Could you check a few things on this model? Use its own coordinates, in mm. A direction names the side the tool comes from. Give positions to 0.01 mm unless a question says otherwise; leave off trailing zeros. Loops run counter-clockwise (first coordinate to the right, second up) from the corner with the lowest first, then second, coordinate; pieces in that order, holes last. Notation, with made-up numbers: (53.25, 47.5) - (71.25, 47.5) arc R27 cw to (71.25, 77.5) - close; hole circle Ø10 at (32, 61.5). An arc over 180 degrees is marked (long way). Use CSV: the item, a comma, the result in double quotes.
from build123d import *

# Parameters (mm, degrees)
SKETCH_R           = 4.25
PAD_DEPTH          = 10
SKETCH001_W        = 16
SKETCH001_H        = 16
POCKET_DEPTH       = 5
FILLET_R           = 7
SKETCH002_W        = 180
SKETCH002_H        = 180
SKETCH002_R        = 57.5
SKETCH002_R_2      = 8
PAD001_DEPTH       = 10
SKETCH003_R        = 58.25
POCKET001_DEPTH    = 20.0010001
SKETCH004_W        = 30
SKETCH004_H        = 30
SKETCH004_R        = 5.5
SKETCH004_R_2      = 1.75
PAD002_DEPTH       = 10
SKETCH005_R        = 12.5
POCKET002_DEPTH    = 5
FILLET001_R        = 14.99
FILLET001_FACE62_R = 4.25
POCKET003_DEPTH    = 10.001
POCKET004_DEPTH    = 10
FILLET002_R        = 7


with BuildPart() as part:
    # Sketch → Pad (new body)
    with BuildSketch(Plane.XY):
        with BuildLine():
            ThreePointArc((0, -57.5), (57.5, 0), (0, 57.5))
            Line((0, 64.5658578507), (0, 57.5))
            Line((-7.5, 64.5658578507), (0, 64.5658578507))
            Line((-7.5, 79.5658578507), (-7.5, 64.5658578507))
            Line((7.5, 79.5658578507), (-7.5, 79.5658578507))
            Line((7.5, 64.5658578507), (7.5, 79.5658578507))
            ThreePointArc((7, -64.6219776856), (64.9995131723, -0.2515697895), (7.5, 64.5658578507))
            Line((7, -64.6219776856), (7, -79.6219776856))
            Line((7, -79.6219776856), (0, -79.6219776856))
            Line((0, -79.6219776856), (0, -57.5))
        make_face()
        with Locations((0, 72.0658578507)):
            Circle(SKETCH_R, mode=Mode.SUBTRACT)
    extrude(amount=PAD_DEPTH)

    # Sketch001 (on Face13 of Pad) → Pocket (cut)
    with BuildSketch(Plane.XY.offset(10)):
        with Locations((-0.5, 72.5)):
            Rectangle(SKETCH001_W, SKETCH001_H)
    extrude(amount=-POCKET_DEPTH, mode=Mode.SUBTRACT)

    # Fillet
    fillet_edges = [part.edges().sort_by_distance(p)[0] for p in [
        (-7.5, 64.565858, 2.5),
        (-7.5, 79.565858, 2.5),
    ]]
    fillet(fillet_edges, radius=FILLET_R)

    # Sketch002 → Pad001 (join)
    with BuildSketch(Plane.XY):
        Rectangle(SKETCH002_W, SKETCH002_H)
        Circle(SKETCH002_R, mode=Mode.SUBTRACT)
        with Locations((75, -75)):
            Circle(SKETCH002_R_2, mode=Mode.SUBTRACT)
        with Locations((75, 75)):
            Circle(SKETCH002_R_2, mode=Mode.SUBTRACT)
        with Locations((-75, 75)):
            Circle(SKETCH002_R_2, mode=Mode.SUBTRACT)
        with Locations((-75, -75)):
            Circle(SKETCH002_R_2, mode=Mode.SUBTRACT)
    extrude(amount=-PAD001_DEPTH)

    # Sketch003 (on Face26 of Pad001) → Pocket001 (cut, through all)
    with BuildSketch(Plane(origin=(0, 0, -10), x_dir=(1, 0, 0), z_dir=(0, 0, -1))):
        Circle(SKETCH003_R)
    extrude(amount=-POCKET001_DEPTH, mode=Mode.SUBTRACT)

    # Sketch004 (on Face2 of Pocket001) → Pad002 (join)
    with BuildSketch(Plane.XY):
        with Locations((0, 105)):
            Rectangle(SKETCH004_W, SKETCH004_H)
        with Locations((0, 105)):
            Circle(SKETCH004_R, mode=Mode.SUBTRACT)
        with Locations((8, 105)):
            Circle(SKETCH004_R_2, mode=Mode.SUBTRACT)
        with Locations((0, 113)):
            Circle(SKETCH004_R_2, mode=Mode.SUBTRACT)
        with Locations((-8, 105)):
            Circle(SKETCH004_R_2, mode=Mode.SUBTRACT)
        with Locations((0, 97)):
            Circle(SKETCH004_R_2, mode=Mode.SUBTRACT)
        with Locations((0, -105)):
            Rectangle(SKETCH004_W, SKETCH004_H)
        with Locations((0, -105)):
            Circle(SKETCH004_R, mode=Mode.SUBTRACT)
        with Locations((8, -105)):
            Circle(SKETCH004_R_2, mode=Mode.SUBTRACT)
        with Locations((0, -97)):
            Circle(SKETCH004_R_2, mode=Mode.SUBTRACT)
        with Locations((-8, -105)):
            Circle(SKETCH004_R_2, mode=Mode.SUBTRACT)
        with Locations((0, -113)):
            Circle(SKETCH004_R_2, mode=Mode.SUBTRACT)
    extrude(amount=-PAD002_DEPTH)

    # Sketch005 (on Face13 of Pad002) → Pocket002 (cut)
    with BuildSketch(Plane.XY):
        with Locations((0, 105)):
            Circle(SKETCH005_R)
        with Locations((0, -105)):
            Circle(SKETCH005_R)
    extrude(amount=-POCKET002_DEPTH, mode=Mode.SUBTRACT)

    # Fillet001
    fillet001_edges = [part.edges().sort_by_distance(p)[0] for p in [
        (15, -120, -5),
        (-15, -120, -5),
        (15, -90, -5),
        (-15, -90, -5),
        (15, 120, -5),
        (-15, 120, -5),
        (15, 90, -5),
        (-15, 90, -5),
        (90, 90, -5),
        (90, -90, -5),
        (-90, -90, -5),
        (-90, 90, -5),
    ]]
    fillet(fillet001_edges, radius=FILLET001_R)

    # Fillet001 Face62 → Pocket003 (cut, through all)
    with BuildSketch(Plane(origin=(0, 72.0658578507, 0), x_dir=(0, 1, 0), z_dir=(0, 0, 1))):
        Circle(FILLET001_FACE62_R)
    extrude(amount=-POCKET003_DEPTH, mode=Mode.SUBTRACT)

    # Sketch006 (on Face56 of Pocket003) → Pocket004 (cut)
    with BuildSketch(Plane.XY.offset(10)):
        with BuildLine():
            ThreePointArc((-25, -60), (0, -65), (25, -60))
            Line((25, -60), (25, -79.1454357496))
            ThreePointArc((-25, -79.1454357496), (0, -83), (25, -79.1454357496))
            Line((-25, -60), (-25, -79.1454357496))
        make_face()
    extrude(amount=-POCKET004_DEPTH, mode=Mode.SUBTRACT)

    # Fillet002
    fillet002_edges = [part.edges().sort_by_distance(p)[0] for p in [
        (7.5, 79.565858, 2.5),
    ]]
    fillet(fillet002_edges, radius=FILLET002_R)


solid = part.part
1) I need wall thicknesses on line 1 along Y through (x, z) = (75, -6.75); line 2 along Y through (x, z) = (0, -0.5); line 3 along Y through (x, z) = (-8, -7.75). Which ranges of each line are inside material? Lowest first, please.
Answer below:
line 1,"y = -90 to -83, -67 to 67, 83 to 90"
line 2,"y = -120 to -117.5, -92.5 to -58.25, 58.25 to 67.82, 76.32 to 92.5, 117.5 to 120"
line 3,"y = -117.69 to -106.75, -103.25 to -57.7, 57.7 to 103.25, 106.75 to 117.69"
2) Which directions (+Z, -Z, +X, -X, +Y, -Y) give clear straight access to the entire face, cutting with the end or side of a thin tool? Please do faces 1 (the cylindrical face through (-5.504, 77.461, 2.535)), 2 (the flat face through (-53, 90, -5)), 3 (the flat face through (0, 61, 5)), 4 (the flat face through (90, -1, -5)).
Answer below:
face 1,"+Z, -X, +Y"
face 2,"+Z, -Z, -X, +Y"
face 3,"+Z, -X, -Y"
face 4,"+Z, -Z, +X, +Y, -Y"
3) I'm going to push flat-ended pins straight in: P1, Ø10, axis at x = 51.5, z = -5.5, coming from the -Y side; P2, Ø3, axis at x = 0, y = -97, coming from the -Z side; P3, Ø10, axis at x = 55, z = 5.5, coming from the -Y side; P4, Ø2, axis at x = -14, z = -6, coming from the +Y side. Where does each tip first touch, or does it pass through?
Answer below:
P1,"stops at y = -90"
P2,"passes through"
P3,"stops at y = -41.53"
P4,"stops at y = 112.49"
4) Suppose I cut it at A-A (y = 0). Please give me the cut outline in (x, z), plus the area to 4 significant figures.
Answer below:
outline,"(-90, -10) - (-58.25, -10) - (-58.25, 0) - (-90, 0) - close; (58.25, -10) - (90, -10) - (90, 0) - (65, 0) - (65, 10) - (58.25, 10) - close"
area,"702.5 mm2"
5) Suppose I cut it at C-C (x = -33). Please give me the cut outline in (y, z).
Answer below:
outline,"(-90, -10) - (-48, -10) - (-48, 0) - (-90, 0) - close; (48, -10) - (90, -10) - (90, 0) - (48, 0) - close"
6) Suppose I cut it at D-D (y = -40). Please give me the cut outline in (x, z), plus the area to 3 significant figures.
Answer below:
outline,"(-90, -10) - (-42.34, -10) - (-42.34, 0) - (-90, 0) - close; (42.34, -10) - (90, -10) - (90, 0) - (51.23, 0) - (51.23, 10) - (42.34, 10) - close"
area,"1,040 mm2"
7) Suppose I cut it at B-B (x = 71). Please give me the cut outline in (y, z).
Answer below:
outline,"(-90, -10) - (-81.93, -10) - (-81.93, 0) - (-90, 0) - close; (-68.07, -10) - (68.07, -10) - (68.07, 0) - (-68.07, 0) - close; (81.93, -10) - (90, -10) - (90, 0) - (81.93, 0) - close"
